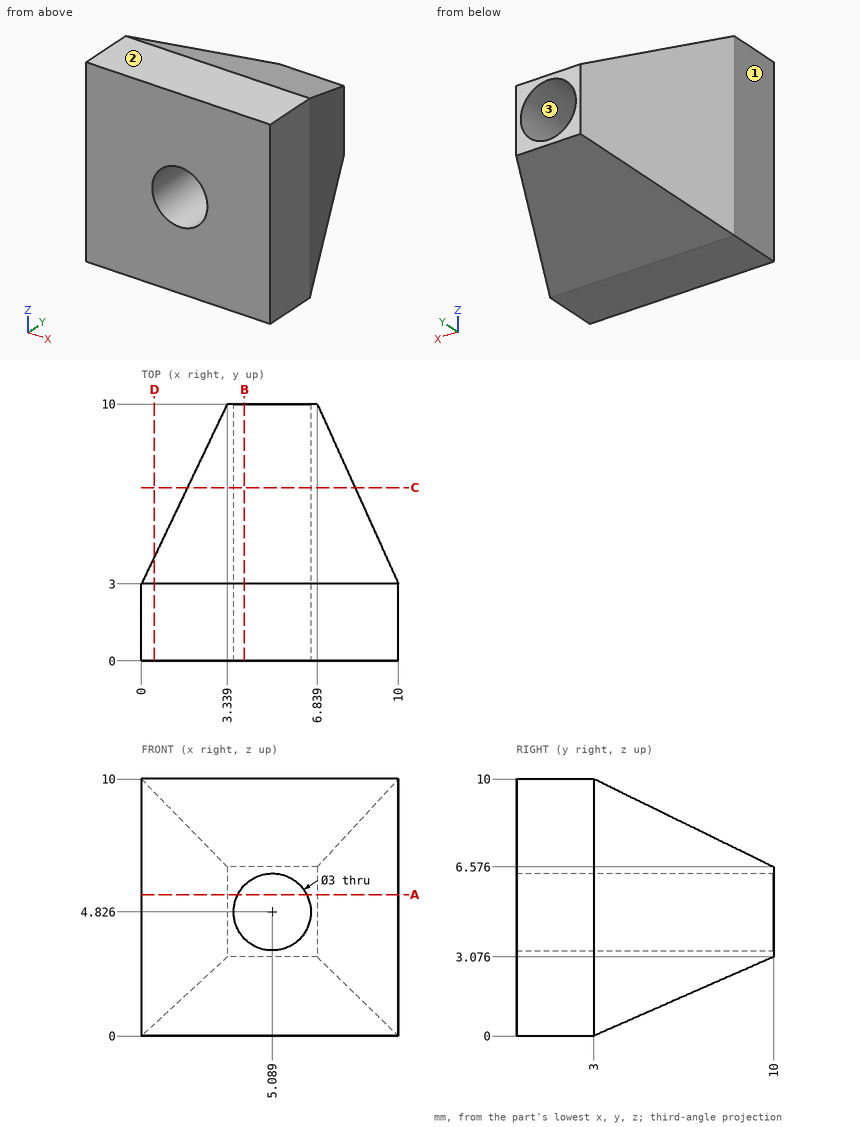
Input: dimensioned drawing with shaded views. Units: mm. Origin: part minimum x, y, z. Round coordinates to 2 decimals unless told otherwise and drop trailing zeros. Order: outer loops, then holes, each group sorted by start corner. A loop starts at its lowest first (then second) coordinate and runs counter-clockwise, first axis right, second up. Notation, with made-up numbers: (87.5, 71.5) - (98.5, 71.5) arc R37 ccw to (98.5, 110.5) - close; hole circle Ø2 at (6, 34). An arc over 180 degrees is marked (long way). Answer as a JSON object with one key per item and string values. Group by question number.
(1) Material intervals for probe 1 along Z at (x, y) = (5.5, 1.75) (1 decimal); probe 2 along X at (y, z) = (9, 4.25) (1 decimal); probe 3 along X at (y, z) = (4.75, 4.25) (1 decimal), sorted ascending. Write a range as from..to.
(2) Pin query (flat end, axial travel): P1, Ø3, axis at y = 7.5, z = 3.5, coming from the -X side; P2, Ø1.5, axis at x = 6, z = 8.5, coming from the +Y side; P3, Ø3, axis at x = 5.5, z = 8.5, coming from the +Y side (1 decimal). Return the tip coordinate at first contact, or that it passes through.
(3) Draft query along Z for the marked faces 1, 2 and 3. Return one class per face: released by +Z, released by -Z, zero draft, split by the parting line, or undercut.
(4) Cut plane C-C (y = 6.75). Return loops of the section in (x, z) (1 decimal).
(5) Cut plane A-A (z = 5.5). Return loops of the section in (x, y).
(6) Cut plane D-D (x = 0.5). Return loops of the section in (y, z).
(7) Cut plane B-B (x = 4). Return loops of the section in (y, z) (1 decimal).
Here are the results:
{
 "1": {"probe 1": "z = 0..3.4, 6.3..10", "probe 2": "x = 2.9..3.7, 6.5..7.3", "probe 3": "x = 0.8..3.7, 6.5..9.2"},
 "2": {"P1": "stops at x = 1.43", "P2": "stops at y = 7.6", "P3": "stops at y = 9.1"},
 "3": {"face 1": "zero draft", "face 2": "released by +Z", "face 3": "undercut"},
 "4": {"outline": "(1.8, 1.6) - (8.3, 1.6) - (8.3, 8.2) - (1.8, 8.2) - close; hole circle Ø3 at (5.1, 4.8)"},
 "5": {"outline": "(0, 0) - (3.75, 0) - (3.75, 10) - (3.34, 10) - (0, 3) - close; (6.43, 0) - (10, 0) - (10, 3) - (6.84, 10) - (6.43, 10) - close"},
 "6": {"outline": "(0, 0) - (3, 0) - (4.05, 0.46) - (4.05, 9.49) - (3, 10) - (0, 10) - close"},
 "7": {"outline": "(0, 0) - (3, 0) - (10, 3.1) - (10, 3.8) - (0, 3.8) - close; (0, 5.9) - (10, 5.9) - (10, 6.6) - (3, 10) - (0, 10) - close"}
}
